Drawing for the job (mm, zero at the part's lowest x, y, z). Give positions to 0.01 mm unless a question says otherwise; leave off trailing zeros. Order: outer loops, then holes, each group sorted by start corner. A loop starts at its lowest first (then second) coordinate and runs counter-clockwise, first axis right, second up. Notation, with made-up numbers: (74, 42) - (126, 42) arc R31 cw to (126, 73) - close; hole circle Ø9 at (-4, 30.25). An arc over 180 degrees is marked (long way). One line per item, written item: value.
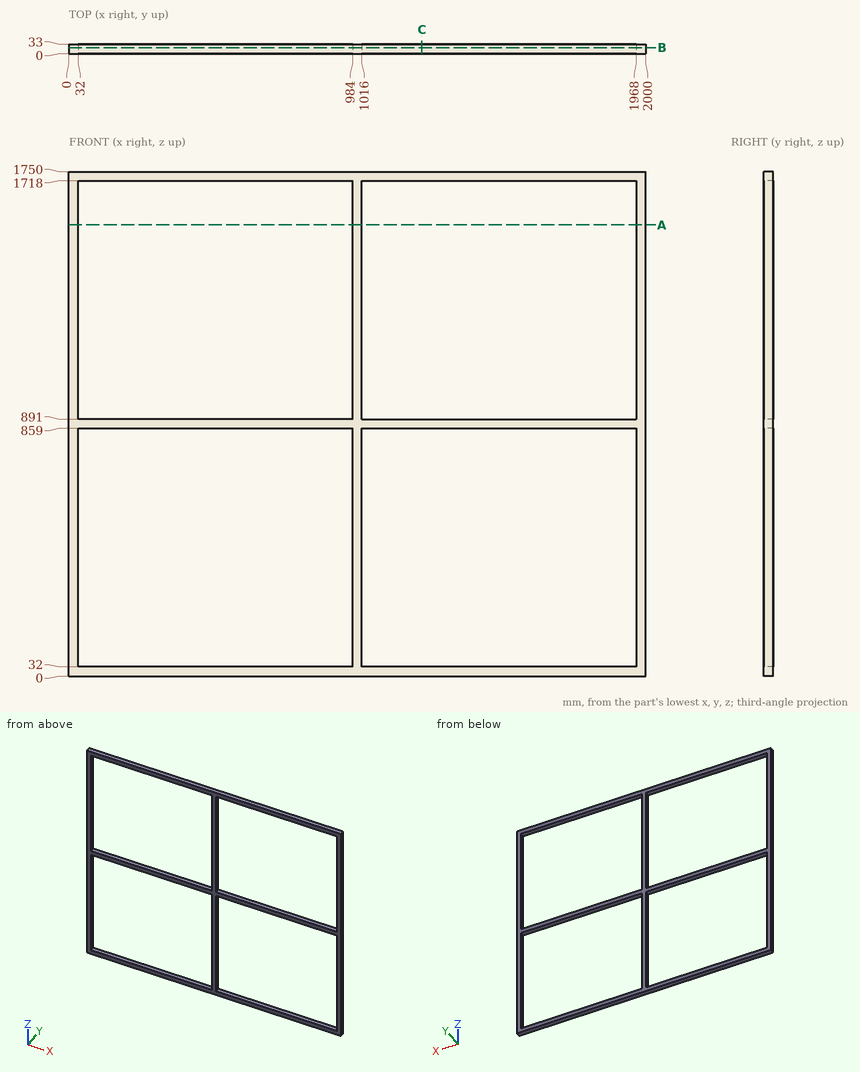
1) Drill centre lines: line 1 along Z through (x, y) = (1861.5, 21.5); line 2 along X through (y, z) = (25, 1654.5). Where is each one in solid material? Low to high. Write a range as from..to.
Outcome:
line 1: z = 0..32, 859..891, 1718..1750
line 2: x = 0..32, 984..1016, 1968..2000
2) Cut at B-B, the plane y = 20.5. Give the cut face in (x, z), then the cut area to 3 significant figures.
Outcome:
outline: (0, 0) - (2000, 0) - (2000, 1750) - (0, 1750) - close; hole (32, 32) - (984, 32) - (984, 859) - (32, 859) - close; hole (32, 891) - (984, 891) - (984, 1718) - (32, 1718) - close; hole (1016, 32) - (1968, 32) - (1968, 859) - (1016, 859) - close; hole (1016, 891) - (1968, 891) - (1968, 1718) - (1016, 1718) - close
area: 351,000 mm^2
3) Cut at C-C, the plane x = 1224. Give the cut face in (y, z).
Outcome:
outline: (0, 0) - (33, 0) - (33, 32) - (0, 32) - close; (0, 859) - (33, 859) - (33, 891) - (0, 891) - close; (0, 1718) - (33, 1718) - (33, 1750) - (0, 1750) - close
4) Cut at A-A, the plane z = 1565. Give the cut face in (x, y), then the cut area to 3 significant figures.
Outcome:
outline: (0, 0) - (32, 0) - (32, 33) - (0, 33) - close; (984, 0) - (1016, 0) - (1016, 33) - (984, 33) - close; (1968, 0) - (2000, 0) - (2000, 33) - (1968, 33) - close
area: 3,170 mm^2
